Build history of the part. All positions in model axes, mm. A direction names the side the tool comes from. Give positions to 0.01 mm unless a question says otherwise; leave off trailing zeros. Loops run counter-clockwise (first coordinate to the right, second up) from the corner with the lowest first, then second, coordinate; pieces in that order, holes last. Notation, with made-up numbers: M 86,66 L 91,66 A21 cw 91,89 Z; hole C -26.5,72 d5. An arc over 180 degrees is marked long. Put each result on its own line as item: value.
```python
from build123d import *

# Parameters (mm, degrees)
BOSS_EXTRUDE1_DEPTH = 21.5
BOSS_EXTRUDE2_DEPTH = 1
SKETCH3_W           = 50
SKETCH3_H           = 20
BOSS_EXTRUDE3_DEPTH = 15
SKETCH8_R           = 1.6
BOSS_EXTRUDE5_DEPTH = 5
SKETCH10_R          = 2.7
SKETCH10_R_2        = 2.6
CUT_EXTRUDE5_DEPTH  = 3
FILLET2_R           = 15
SKETCH11_W          = 43.237900078
SKETCH11_H          = 3
CUT_EXTRUDE7_DEPTH  = 20


with BuildPart() as part:
    # Sketch1 → Boss-Extrude1 (new body)
    with BuildSketch(Plane.XY):
        with BuildLine():
            Line((71, 0), (70, 0))
            ThreePointArc((70, 0), (0, -70), (-70, 0))
            Line((-70, 0), (-71, 0))
            ThreePointArc((-71, 0), (0, -71), (71, 0))
        make_face()
    extrude(amount=BOSS_EXTRUDE1_DEPTH)

    # Sketch2 → Boss-Extrude2 (add)
    with BuildSketch(Plane.XY.offset(21.5)):
        with BuildLine():
            Line((71, 0), (70, 0))
            ThreePointArc((70, 0), (0, -70), (-70, 0))
            Line((-70, 0), (-71, 0))
            ThreePointArc((-71, 0), (0, -71), (71, 0))
        make_face()
        with BuildLine():
            Line((-42, 0), (-70, 0))
            ThreePointArc((-70, 0), (0, -70), (70, 0))
            Line((70, 0), (42, 0))
            ThreePointArc((42, 0), (0, -42), (-42, 0))
        make_face()
    extrude(amount=BOSS_EXTRUDE2_DEPTH)

    # Sketch3 → Boss-Extrude3 (add)
    with BuildSketch(Plane(origin=(0, 0, 0), x_dir=(-1, 0, 0), z_dir=(0, 0, -1))):
        with BuildLine():
            Line((-25, -66.452990903), (-25, -71))
            Line((-25, -71), (0, -71))
            ThreePointArc((0, -71), (-12.705070757, -69.853999006), (-25, -66.452990903))
        make_face()
        with BuildLine():
            ThreePointArc((25, -66.452990903), (12.705070757, -69.853999006), (0, -71))
            Line((0, -71), (25, -71))
            Line((25, -71), (25, -66.452990903))
        make_face()
        with Locations((0, -81)):
            Rectangle(SKETCH3_W, SKETCH3_H)
    extrude(amount=-BOSS_EXTRUDE3_DEPTH)

    # Sketch8 → Boss-Extrude5 (add)
    # profile 1 of 2: a face of its own
    with BuildSketch(Plane(origin=(0, 0, 0), x_dir=(-1, 0, 0), z_dir=(0, 0, -1))):
        with BuildLine():
            ThreePointArc((-70.654086931, -7), (-70.913469003, -3.504270818), (-71, 0))
            Line((-71, 0), (-78, 0))
            Line((-78, 0), (-78, -7))
            Line((-78, -7), (-70.654086931, -7))
        make_face()
        with Locations((-74.5, -3.5)):
            Circle(SKETCH8_R, mode=Mode.SUBTRACT)
    # profile 2 of 2: a face of its own
    with BuildSketch(Plane(origin=(0, 0, 0), x_dir=(-1, 0, 0), z_dir=(0, 0, -1))):
        with BuildLine():
            Line((78, 0), (71, 0))
            ThreePointArc((71, 0), (70.913469003, -3.504270818), (70.654086931, -7))
            Line((70.654086931, -7), (78, -7))
            Line((78, -7), (78, 0))
        make_face()
        with Locations(Location((74.5, -3.5, 0), (0, 0, 180))):
            Circle(SKETCH8_R, mode=Mode.SUBTRACT)
    extrude(amount=-BOSS_EXTRUDE5_DEPTH)

    # Sketch10 → Cut-Extrude5 (cut)
    with BuildSketch(Plane.XY.offset(5)):
        with Locations((74.5, -3.5)):
            Circle(SKETCH10_R)
        with Locations((-74.5, -3.5)):
            Circle(SKETCH10_R_2)
    extrude(amount=-CUT_EXTRUDE5_DEPTH, mode=Mode.SUBTRACT)

    # Fillet2
    fillet2_edges = [part.edges().sort_by_distance(p)[0] for p in [
        (-25, -78.726495452, 15),
        (25, -78.726495452, 15),
    ]]
    fillet(fillet2_edges, radius=FILLET2_R - 0.0001)  # a hair under: the kernel refuses the full size

    # Sketch11 → Cut-Extrude7 (cut)
    with BuildSketch(Plane.XZ.offset(91)):
        with Locations((0, 1.5)):
            Rectangle(SKETCH11_W, SKETCH11_H)
        with BuildLine():
            Line((-21.618950039, 3), (21.618950039, 3))
            ThreePointArc((21.618950039, 3), (17.348469228, 9.486832981), (10, 12))
            Line((10, 12), (-10, 12))
            ThreePointArc((-10, 12), (-17.348469228, 9.486832981), (-21.618950039, 3))
        make_face()
    extrude(amount=-CUT_EXTRUDE7_DEPTH, mode=Mode.SUBTRACT)


solid = part.part
```
Q1. Slice it at B-B (y = -62.5). List the corners of the cut face in (x, z), and give its area (3 significant figures).
Here are the results:
outline: M -33.69,0 L -31.52,0 L -31.52,21.5 L 31.52,21.5 L 31.52,0 L 33.69,0 L 33.69,22.5 L -33.69,22.5 Z
area: 160 mm²
Q2. Drop flat-ended pins along their axis: pin 1 Ø1.5 at (y, z) = (-83.5, 2) entering from -X; pin 2 Ø3 at (x, y) = (-3.5, -50.5) entering from -Z; pin 3 Ø2.5 at (x, z) = (-73.5, 3) entering from -Y. Give the stop position or say it passes through.
Here are the results:
pin 1: x = -24.95
pin 2: z = 21.5
pin 3: y = -7
Q3. Slice it at D-D (x = 0). List the corners of the cut face in (y, z), and give its area (4 significant figures).
Here are the results:
outline: M -91,12 L -71,12 L -71,0 L -70,0 L -70,21.5 L -42,21.5 L -42,22.5 L -71,22.5 L -71,15 L -91,15 Z
area: 110.5 mm²
Q4. Tool access for faces 3 (the cylindrical face through (17.436, -81.14, 9.419)), 4 (the cylindrical face through (-77.1, -3.4, 3.5)), 5 (the flat face through (-74, -7, 2)): list every direction of +Z, -Z, +X, -X, +Y, -Y with a clear straight run to the whole face (end or side of a thin tool).
Here are the results:
face 3: -Z, -Y
face 4: +Z
face 5: +Z, -Z, -X, -Y
Q5. Slice it at A-A (x = 74.5). List the corners of the cut face in (y, z).
Here are the results:
outline: M -7,0 L -5.1,0 L -5.1,2 L -6.2,2 L -6.2,5 L -7,5 Z; M -1.9,0 L 0,0 L 0,5 L -0.8,5 L -0.8,2 L -1.9,2 Z
Q6. Slice it at C-C (z = 7). List the corners of the cut face in (x, y).
Here are the results:
outline: M -71,0 A71 ccw -23.27,-67.08 L -23.27,-91 L -19.75,-91 L -19.75,-71 L 19.75,-71 L 19.75,-91 L 23.27,-91 L 23.27,-67.08 A71 ccw 71,0 L 70,0 A70 cw -70,0 Z
Q7. Mould opens along X. For faces 1 (the flat face through (-17, -69, 0)), 2 (the flat face through (0, -81, 12)) say: pulls with the +X half, pulls with the -X half, needs draft (parallel to the pull), parting line crosses it, or undercut.
Here are the results:
face 1: needs draft
face 2: undercut
Q8. Probe line 1 (Y direction, x = 74.5, z = 4); line 2 (Y direction, x = 74.5, z = 1.35); line 3 (Z direction, x = -1, y = -63). List the from-to ranges inside material, lowest first. Write a range as from..to.
Here are the results:
line 1: -7..-6.2, -0.8..0
line 2: -7..-5.1, -1.9..0
line 3: 21.5..22.5
